Work out the finished part from the listing and answer in its coordinate system (mm). A direction names the side the tool comes from. Round coordinates to 2 decimals unless told otherwise and drop trailing zeros. Order: outer loops, then holes, each group sorted by start corner. A loop starts at its lowest first (then second) coordinate and runs counter-clockwise, first axis right, second up. Notation, with made-up numbers: (45.25, -34.5) -> (51.25, -34.5) arc R19 ccw to (51.25, 2.5) -> close; hole circle Ø4 at (-3.5, -14.75). An arc over 180 degrees is marked (long way). Use one line per item in the form item = value.
Autodesk Inventor part; units mm, degrees
ref_plane "YZ Plane" through (0, 0, 0) normal (1, 0, 0) x (0, 1, 0)
ref_plane "XZ Plane" through (0, 0, 0) normal (0, 1, 0) x (-1, 0, 0)
ref_plane "XY Plane" through (0, 0, 0) normal (0, 0, 1) x (1, 0, 0)
sketch "Sketch1" plane through (0, 0, 0) normal (0, 1, 0) x (-1, 0, 0)
  line L0 (0, 0) -> (-98, 0)
  line L1 (-98, 0) -> (-98, -100)
  line L2 (-98, -100) -> (0, -100)
  line L3 (0, -100) -> (0, 0)
  line L4 (3, -103) -> (-101, -103)
  line L5 (-101, -103) -> (-101, 3)
  line L6 (-101, 3) -> (3, 3)
  line L7 (3, 3) -> (3, -103)
  line L8 (0, -20) -> (-6, -20)
  line L9 (-6, -20) -> (-6, -80)
  line L10 (-6, -80) -> (0, -80)
  line L11 (0, -80) -> (0, -20)
  line L12 (-46, -20) -> (-52, -20)
  line L13 (-52, -20) -> (-52, -80)
  line L14 (-52, -80) -> (-46, -80)
  line L15 (-46, -80) -> (-46, -20)
  line L16 (-92, -20) -> (-98, -20)
  line L17 (-98, -20) -> (-98, -80)
  line L18 (-98, -80) -> (-92, -80)
  line L19 (-92, -80) -> (-92, -20)
  point P0 (-49, -20)
  point P1 (-6, -50)
  point P2 (-98, -20)
  point P3 (-98, -80)
  point P4 (0, -80)
  point P5 (0, -20)
  dimension "d0" = 100
  dimension "d1" = 98
  dimension "d2" = 3
  dimension "d48" = 6
  dimension "d49" = 60
  dimension "d50" = 6
  dimension "d51" = 60
  dimension "d52" = 6
  dimension "d53" = 60
  dimension "d54" = 49
  dimension "d55" = 50
extrude "Extrusion1" add sketch "Sketch1" along normal blind 4 contours L3 L8 L9 L10 L2 L1 L18 L19 L16 L0 | L3 L10 L9 L8 | L16 L19 L18 L1 | L15 L14 L13 L12
extrude "Extrusion2" add sketch "Sketch1" along normal blind 55 contours L4 L5 L6 L7
fillet "Fillet1" radius 2 4 edges at (-3, 27.5, 3) (101, 27.5, 3) (101, 27.5, -103) (-3, 27.5, -103)
sketch "Sketch2" plane through (0, 4, 0) normal (0, 1, 0) x (1, 0, 0)
  line L0 (98, 0) -> (98, 100)
  line L1 (98, 100) -> (0, 100)
  line L2 (0, 100) -> (0, 0)
  line L3 (0, 0) -> (98, 0)
  circle A0 centre (5.185, 73.913) radius 3
  circle A1 centre (5.185, 6.858) radius 3
  circle A2 centre (92.815, 6.858) radius 3
  circle A3 centre (92.815, 73.913) radius 3
  dimension "d8" = 6
  dimension "d9" = 6
  dimension "d10" = 6
  dimension "d11" = 6
  dimension "d12" = 67.055
  dimension "d13" = 87.63
  dimension "d16" = 6.858
  dimension "d17" = 5.185
extrude "Extrusion3" add sketch "Sketch2" along normal blind 19 contours A0 | A1 | A2 | A3
sketch "Sketch3" plane through (92.815, 23, -73.913) normal (0, 1, 0) x (1, 0, 0)
  circle A0 centre (0, -67.055) radius 3
  circle A1 centre (0, -67.055) radius 0.75
  circle A2 centre (0, 0) radius 3
  circle A3 centre (0, 0) radius 0.75
  circle A4 centre (-87.63, 0) radius 3
  circle A5 centre (-87.63, 0) radius 0.75
  circle A6 centre (-87.63, -67.055) radius 3
  circle A7 centre (-87.63, -67.055) radius 0.75
  point P0 (-92.815, -73.913)
  dimension "d21" = 1.5
  dimension "d22" = 1.5
  dimension "d23" = 1.5
  dimension "d24" = 1.5
extrude "Extrusion4" cut sketch "Sketch3" against normal blind 5 contours A1 | A3 | A5 | A7
fillet "Fillet2" radius 2 4 edges at (89.815, 4, -73.913) (89.815, 4, -6.858) (2.185, 4, -6.858) (2.185, 4, -73.913)
extrude "Extrusion5" cut sketch "Sketch1" along normal blind 2 contours L3 L10 L9 L8 | L16 L19 L18 L1 | L15 L14 L13 L12
sketch "Sketch4" plane through (-1, 0, 3) normal (0, 0, 1) x (1, 0, 0)
  line L0 (11.185, 4) -> (1.185, 4)
  line L1 (98.815, 4) -> (88.815, 4)
  line L2 (99, 4) -> (1, 4)
  line L3 (1, 4) -> (99, 4)
  line L4 (98.815, 4) -> (88.815, 4)
  line L5 (11.185, 4) -> (1.185, 4)
  line L6 (1, 4) -> (1, 55)
  line L7 (1, 4) -> (1, 55)
  line L8 (99, 4) -> (99, 55)
  line L9 (99, 4) -> (99, 55)
  line L10 (43.14, 49.31) -> (32.39, 49.31)
  line L11 (32.39, 49.31) -> (32.39, 37.21)
  line L12 (32.39, 37.21) -> (43.14, 37.21)
  line L13 (43.14, 37.21) -> (43.14, 49.31)
  line L14 (49.815, 5.39) -> (59.815, 5.39)
  line L15 (59.815, 5.39) -> (59.815, 10.39)
  line L16 (59.815, 10.39) -> (49.815, 10.39)
  line L17 (49.815, 10.39) -> (49.815, 5.39)
  line L18 (62.14, 49.31) -> (70.89, 49.31)
  line L19 (70.89, 49.31) -> (70.89, 37.21)
  line L20 (70.89, 37.21) -> (62.14, 37.21)
  line L21 (62.14, 37.21) -> (62.14, 49.31)
  line L22 (9.185, 23) -> (3.185, 23)
  line L23 (96.815, 23) -> (90.815, 23)
  circle A0 centre (13.6833, 36.5386) radius 2.5
  circle A1 centre (22.8325, 36.5386) radius 2.5
  circle A2 centre (88.2047, 36.5386) radius 2.5
  point P0 (1, 0)
  point P1 (66.515, 37.21)
  point P2 (70.89, 43.26)
  point P3 (59.815, 7.89)
  point P4 (49.815, 7.89)
  point P5 (54.815, 5.39)
  point P6 (54.815, 10.39)
  point P7 (6.185, 23)
  point P8 (37.765, 37.21)
  point P9 (93.815, 23)
  dimension "d56" = 12.1
  dimension "d57" = 19
  dimension "d59" = 10.75
  dimension "d60" = 12.1
  dimension "d61" = 8.75
  dimension "d62" = 10
  dimension "d63" = 5
  dimension "d103" = 12.61
  dimension "d105" = 14.21
  dimension "d106" = 39
  dimension "d107" = 27.3
  dimension "d108" = 5
  dimension "d109" = 5
  dimension "d110" = 5
extrude "Extrusion6" cut sketch "Sketch4" against normal up to surface (3 mm away)
sketch "Sketch5" plane through (101, 0, 1) normal (1, 0, 0) x (0, 0, -1)
  line L0 (12.858, 4) -> (2.858, 4)
  line L1 (79.913, 4) -> (69.913, 4)
  line L2 (1, 4) -> (101, 4)
  line L3 (101, 4) -> (1, 4)
  line L4 (12.858, 4) -> (2.858, 4)
  line L5 (79.913, 4) -> (69.913, 4)
  line L6 (1, 37.21) -> (1, 49.31)
  line L7 (1, 49.31) -> (1, 37.21)
  line L8 (1, 49.31) -> (1, 37.21)
  line L9 (1, 37.21) -> (1, 49.31)
  line L10 (1, 4) -> (1, 55)
  line L11 (1, 4) -> (1, 55)
  line L12 (10.858, 23) -> (4.858, 23)
  line L13 (77.913, 23) -> (71.913, 23)
  line L14 (18.133, 24.6) -> (69.133, 24.6)
  line L15 (69.133, 24.6) -> (69.133, 34.6)
  line L16 (69.133, 34.6) -> (18.133, 34.6)
  line L17 (18.133, 34.6) -> (18.133, 24.6)
  line L18 (12.858, 4) -> (2.858, 4)
  line L19 (4.858, 6) -> (10.858, 6)
  line L20 (79.913, 4) -> (69.913, 4)
  line L21 (71.913, 6) -> (77.913, 6)
  line L22 (1, 10.39) -> (1, 5.39)
  line L23 (1, 5.39) -> (1, 10.39)
  point P0 (1, 0)
  point P1 (74.913, 23)
  dimension "d98" = 10
  dimension "d99" = 51
  dimension "d101" = 1.6
  dimension "d102" = 5.78
sketch "Sketch6" plane through (-3, 0, -101) normal (-1, 0, 0) x (0, 0, 1)
  line L0 (32.867, 34.6) -> (83.867, 34.6)
  line L1 (32.867, 24.6) -> (32.867, 34.6)
  line L2 (83.867, 24.6) -> (32.867, 24.6)
  line L3 (83.867, 34.6) -> (83.867, 24.6)
  point P0 (101, 0)
extrude "Extrusion7" cut sketch "Sketch5" against normal up to surface (3 mm away)
extrude "Extrusion8" cut sketch "Sketch6" against normal up to surface (3 mm away)
sketch "Sketch7" plane through (0, 55, 0) normal (0, 1, 0) x (1, 0, 0)
  circle A0 centre (-1.2, -1.2) radius 0.8
  circle A1 centre (99.2, -1.2) radius 0.8
  line L0 (98, 100) -> (98, 0)
  circle A2 centre (99.2, 101.2) radius 0.8
  line L1 (0, 100) -> (98, 100)
  circle A3 centre (-1.2, 101.2) radius 0.8
  line L2 (0, 0) -> (0, 100)
  circle A4 centre (32.27, -1.2) radius 0.8
  circle A5 centre (32.27, 101.2) radius 0.8
  circle A6 centre (65.74, -1.2) radius 0.8
  circle A7 centre (65.74, 101.2) radius 0.8
  circle A8 centre (-1.2, 36.27) radius 0.8
  circle A9 centre (99.2, 36.27) radius 0.8
  circle A10 centre (-1.2, 73.74) radius 0.8
  circle A11 centre (99.2, 73.74) radius 0.8
  dimension "d1" = 98
  dimension "d64" = 1.6
  dimension "d65" = 1.2
  dimension "d66" = 1.2
  dimension "d67" = 1.6
  dimension "d68" = 1.2
  dimension "d69" = 1.6
  dimension "d70" = 1.2
  dimension "d71" = 1.2
  dimension "d72" = 1.6
  dimension "d73" = 1.2
  dimension "d74" = 1.2
  dimension "d87" = 33.47
  dimension "d91" = 37.47
extrude "Extrusion9" cut sketch "Sketch7" against normal blind 0.8
properties part number "Base Chassis"
Item 1: The part is cut by section B-B, the plane x = 82. Give the vertices of the cut face in (y, z), and give its area (3 significant figures).
Findings:
outline = (0, -103) -> (55, -103) -> (55, -100) -> (4, -100) -> (4, 0) -> (55, 0) -> (55, 3) -> (0, 3) -> close
area = 730 mm^2
Item 2: For faces 4 (the flat face through (-2, 34.6, -43)), 5 (the flat face through (49, 2, -50)), 6 (the flat face through (37, 49.31, 2)), 7 (the flat face through (98, 35, -49)), determine the directions among +Z, -Z, +X, -X, +Y, -Y from which every point of the face is accessible in a straight line to the end or side of a thin tool.
Findings:
face_4 = +X, -X
face_5 = -Y
face_6 = +Z
face_7 = +Y
Item 3: The part is cut by section D-D, the plane z = -92. Give the vertices of the cut face in (x, y).
Findings:
outline = (-3, 0) -> (101, 0) -> (101, 55) -> (98, 55) -> (98, 4) -> (0, 4) -> (0, 55) -> (-3, 55) -> close
Item 4: Determine the mould class of faces 1 (the flat face through (54, 5.39, 2)), 2 (the flat face through (93, 23, -8)), 3 (the cylindrical face through (4.79, 14.38, -70.94)) for opening direction Y: released by +Y, released by -Y, zero draft, split by the parting line, or undercut.
Findings:
face_1 = undercut
face_2 = released by +Y
face_3 = zero draft
Item 5: Consider line 1 along Z through (x, y) = (-1.2, 54.6); line 2 along X through (y, z) = (54.7, -73.74); line 3 along Z through (x, y) = (65.74, 54.45). Determine where each line is inside the solid, lowest interval first.
Findings:
line_1 = -102.99 to -102, -100.4 to -74.54, -72.94 to -37.07, -35.47 to 0.4, 2 to 2.99
line_2 = -3 to -2, -0.4 to 0, 98 to 98.4, 100 to 101
line_3 = -103 to -102, -100.4 to -100, 0 to 0.4, 2 to 3
Item 6: Flat-ended cylindrical pins translate along their axes: P1, Ø6.5, axis at x = 6, z = -73, coming from the +Y side; P2, Ø0.9, axis at y = 7.5, z = 2, coming from the +X side; P3, Ø5, axis at x = 28, z = -86, coming from the +Y side. Find the tip coordinate at first contact, or state that the pin passes through.
Findings:
P1 = 23
P2 = 100.92
P3 = 4
Item 7: The part is cut by section C-C, the plane z = -60. Give the vertices of the cut face in (x, y).
Findings:
outline = (-3, 0) -> (0, 0) -> (0, 2) -> (6, 2) -> (6, 0) -> (46, 0) -> (46, 2) -> (52, 2) -> (52, 0) -> (92, 0) -> (92, 2) -> (98, 2) -> (98, 0) -> (101, 0) -> (101, 24.6) -> (98, 24.6) -> (98, 4) -> (0, 4) -> (0, 24.6) -> (-3, 24.6) -> close; (-3, 34.6) -> (0, 34.6) -> (0, 55) -> (-3, 55) -> close; (98, 34.6) -> (101, 34.6) -> (101, 55) -> (98, 55) -> close
Item 8: The part is cut by section A-A, the plane y = 46. Give the vertices of the cut face in (x, z), and give its area (3 significant figures).
Findings:
outline = (-3, -101) arc R2 ccw to (-1, -103) -> (99, -103) arc R2 ccw to (101, -101) -> (101, 1) arc R2 ccw to (99, 3) -> (69.89, 3) -> (69.89, 0) -> (98, 0) -> (98, -100) -> (0, -100) -> (0, 0) -> (31.39, 0) -> (31.39, 3) -> (-1, 3) arc R2 ccw to (-3, 1) -> close; (42.14, 0) -> (61.14, 0) -> (61.14, 3) -> (42.14, 3) -> close
area = 1,160 mm^2
